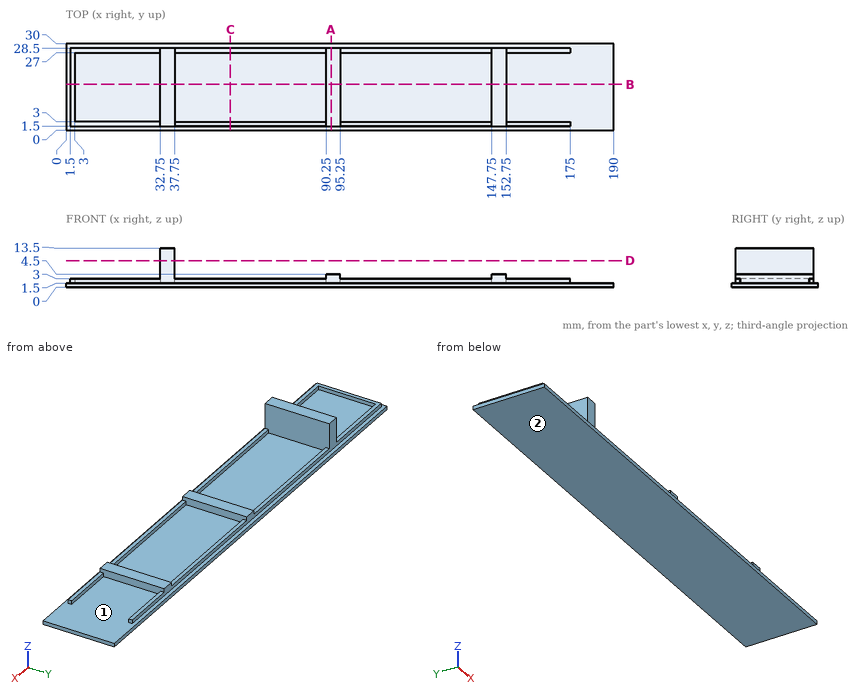
Answer from the drawing. Dimensions are ordinates in mm from the lowest x, y and z of the part. Coordinates: 2 decimals unless noted, no trailing zeros. Loops run counter-clockwise (first coordinate to the right, second up) from the corner with the lowest first, then second, coordinate; pieces in that order, holes last. Notation, with made-up numbers: (-1, 84) -> (30, 84) arc R35 ccw to (30, 119) -> close; hole circle Ø10 at (44, 79). An arc over 180 degrees is marked (long way). Answer in a Markdown table with one row per item.
Item 1: A cutting plane is placed at C-C on x = 57. Determine the outline of the cut face in (y, z).
Returned:
| item | result |
|---|---|
| outline | (0, 0) -> (30, 0) -> (30, 1.5) -> (28.5, 1.5) -> (28.5, 3) -> (27, 3) -> (27, 1.5) -> (3, 1.5) -> (3, 3) -> (1.5, 3) -> (1.5, 1.5) -> (0, 1.5) -> close |
Item 2: Each of these flat-tipped pins is pushed along its axis until it touches: P1, Ø0.8, axis at x = 69.5, z = 2, coming from the +Y side; P2, Ø1.6, axis at y = 27.5, z = 2.5, coming from the +X side; P3, Ø0.8, axis at x = 111.5, z = 2, coming from the -Y side. Where does it stop, or does it pass through?
Returned:
| item | result |
|---|---|
| P1 | stops at y = 28.5 |
| P2 | stops at x = 175 |
| P3 | stops at y = 1.5 |
Item 3: A cutting plane is placed at D-D on z = 9.25. Determine the outline of the cut face in (x, y).
Returned:
| item | result |
|---|---|
| outline | (32.75, 1.5) -> (37.75, 1.5) -> (37.75, 28.5) -> (32.75, 28.5) -> close |
Item 4: A cutting plane is placed at B-B on y = 16. Determine the outline of the cut face in (x, z), plus the area to 3 significant figures.
Returned:
| item | result |
|---|---|
| outline | (0, 0) -> (190, 0) -> (190, 1.5) -> (152.75, 1.5) -> (152.75, 4.5) -> (147.75, 4.5) -> (147.75, 1.5) -> (95.25, 1.5) -> (95.25, 4.5) -> (90.25, 4.5) -> (90.25, 1.5) -> (37.75, 1.5) -> (37.75, 13.5) -> (32.75, 13.5) -> (32.75, 1.5) -> (3, 1.5) -> (3, 3) -> (1.5, 3) -> (1.5, 1.5) -> (0, 1.5) -> close |
| area | 377 mm^2 |
Item 5: Straight lines are drawn through the part: line 1 along X through (y, z) = (24, 3.5); line 2 along X through (y, z) = (4.25, 2.75); line 3 along Z through (x, y) = (135, 14). For each, find the intervals that lie inside material, in ascending order. Write a range as [from, to].
Returned:
| item | result |
|---|---|
| line 1 | x = [32.75, 37.75], [90.25, 95.25], [147.75, 152.75] |
| line 2 | x = [1.5, 3], [32.75, 37.75], [90.25, 95.25], [147.75, 152.75] |
| line 3 | z = [0, 1.5] |
Item 6: A cutting plane is placed at A-A on x = 92. Determine the outline of the cut face in (y, z), plus the area to 3 significant figures.
Returned:
| item | result |
|---|---|
| outline | (0, 0) -> (30, 0) -> (30, 1.5) -> (28.5, 1.5) -> (28.5, 4.5) -> (1.5, 4.5) -> (1.5, 1.5) -> (0, 1.5) -> close |
| area | 126 mm^2 |
Item 7: For a pull along Y with two mould halves and no side action, classify the marked faces 1 and 2 as released by +Y, released by -Y, zero draft, split by the parting line, or undercut.
Returned:
| item | result |
|---|---|
| face 1 | undercut |
| face 2 | zero draft |
